from build123d import *

# Parameters (mm, degrees)
ESQUISSE2_W             = 35
ESQUISSE2_H             = 40
BOSS_EXTRU_1_DEPTH      = 5
ESQUISSE3_W             = 63
ESQUISSE3_H             = 38
BOSS_EXTRU_2_DEPTH      = 2.5
ENL_V_MAT_EXTRU_1_REACH = 58.932
ESQUISSE4_R             = 2
ENL_V_MAT_EXTRU_2_REACH = 58.932
ESQUISSE5_W             = 7
ESQUISSE5_H             = 18
CONG_1_R                = 2
CONG_2_R                = 5
CONG_3_R                = 2
ENL_V_MAT_EXTRU_3_REACH = 54.369
ESQUISSE6_R             = 2


with BuildPart() as part:
    # Esquisse2 → Boss.-Extru.1 (new body)
    with BuildSketch(Plane(origin=(0, 0, 0), x_dir=(1, 0, 0), z_dir=(0, 1, 0))):
        Rectangle(ESQUISSE2_W, ESQUISSE2_H)
    extrude(amount=BOSS_EXTRU_1_DEPTH)

    # Esquisse3 → Boss.-Extru.2 (add, symmetric)
    with BuildSketch(Plane(origin=(0, 0, 0), x_dir=(0, 0, -1), z_dir=(1, 0, 0))):
        with Locations((0, 24)):
            Rectangle(ESQUISSE3_W, ESQUISSE3_H)
    extrude(amount=BOSS_EXTRU_2_DEPTH, both=True)

    # Esquisse4 → Enlèv. mat.-Extru.1 (cut, up to next)
    with BuildSketch(Plane(origin=(2.5, 0, 0), x_dir=(0, 0, -1), z_dir=(1, 0, 0)), mode=Mode.PRIVATE) as enl_v_mat_extru_1_sk1:
        with Locations((-27.94, 37.97)):
            Circle(ESQUISSE4_R)
    enl_v_mat_extru_1_tool1 = extrude(enl_v_mat_extru_1_sk1.sketch, amount=-ENL_V_MAT_EXTRU_1_REACH, mode=Mode.PRIVATE) & part.part
    # Esquisse4 → Enlèv. mat.-Extru.1 (cut, up to next)
    with BuildSketch(Plane(origin=(2.5, 0, 0), x_dir=(0, 0, -1), z_dir=(1, 0, 0)), mode=Mode.PRIVATE) as enl_v_mat_extru_1_sk2:
        with Locations((-27.94, 10.03)):
            Circle(ESQUISSE4_R)
    enl_v_mat_extru_1_tool2 = extrude(enl_v_mat_extru_1_sk2.sketch, amount=-ENL_V_MAT_EXTRU_1_REACH, mode=Mode.PRIVATE) & part.part
    # Esquisse4 → Enlèv. mat.-Extru.1 (cut, up to next)
    with BuildSketch(Plane(origin=(2.5, 0, 0), x_dir=(0, 0, -1), z_dir=(1, 0, 0)), mode=Mode.PRIVATE) as enl_v_mat_extru_1_sk3:
        with Locations((27.94, 37.97)):
            Circle(ESQUISSE4_R)
    enl_v_mat_extru_1_tool3 = extrude(enl_v_mat_extru_1_sk3.sketch, amount=-ENL_V_MAT_EXTRU_1_REACH, mode=Mode.PRIVATE) & part.part
    # Esquisse4 → Enlèv. mat.-Extru.1 (cut, up to next)
    with BuildSketch(Plane(origin=(2.5, 0, 0), x_dir=(0, 0, -1), z_dir=(1, 0, 0)), mode=Mode.PRIVATE) as enl_v_mat_extru_1_sk4:
        with Locations((27.94, 10.03)):
            Circle(ESQUISSE4_R)
    enl_v_mat_extru_1_tool4 = extrude(enl_v_mat_extru_1_sk4.sketch, amount=-ENL_V_MAT_EXTRU_1_REACH, mode=Mode.PRIVATE) & part.part
    add(enl_v_mat_extru_1_tool1.solids().sort_by_distance((2.5, 37.97, 27.94))[0], mode=Mode.SUBTRACT)
    add(enl_v_mat_extru_1_tool2.solids().sort_by_distance((2.5, 10.03, 27.94))[0], mode=Mode.SUBTRACT)
    add(enl_v_mat_extru_1_tool3.solids().sort_by_distance((2.5, 37.97, -27.94))[0], mode=Mode.SUBTRACT)
    add(enl_v_mat_extru_1_tool4.solids().sort_by_distance((2.5, 10.03, -27.94))[0], mode=Mode.SUBTRACT)

    # Esquisse5 → Enlèv. mat.-Extru.2 (cut, up to next)
    with BuildSketch(Plane(origin=(2.5, 0, 0), x_dir=(0, 0, -1), z_dir=(1, 0, 0)), mode=Mode.PRIVATE) as enl_v_mat_extru_2_sk1:
        with Locations((-28, 24)):
            Rectangle(ESQUISSE5_W, ESQUISSE5_H)
    enl_v_mat_extru_2_tool1 = extrude(enl_v_mat_extru_2_sk1.sketch, amount=-ENL_V_MAT_EXTRU_2_REACH, mode=Mode.PRIVATE) & part.part
    # Esquisse5 → Enlèv. mat.-Extru.2 (cut, up to next)
    with BuildSketch(Plane(origin=(2.5, 0, 0), x_dir=(0, 0, -1), z_dir=(1, 0, 0)), mode=Mode.PRIVATE) as enl_v_mat_extru_2_sk2:
        with Locations((28, 24)):
            Rectangle(ESQUISSE5_W, ESQUISSE5_H)
    enl_v_mat_extru_2_tool2 = extrude(enl_v_mat_extru_2_sk2.sketch, amount=-ENL_V_MAT_EXTRU_2_REACH, mode=Mode.PRIVATE) & part.part
    add(enl_v_mat_extru_2_tool1.solids().sort_by_distance((2.5, 24, 28))[0], mode=Mode.SUBTRACT)
    add(enl_v_mat_extru_2_tool2.solids().sort_by_distance((2.5, 24, -28))[0], mode=Mode.SUBTRACT)

    # Congé1
    cong_1_edges = [part.edges().sort_by_distance(p)[0] for p in [
        (0, 15, -24.5),
        (0, 33, -24.5),
        (0, 15, 24.5),
        (0, 33, 24.5),
        (-2.5, 5, 0),
        (2.5, 5, 0),
    ]]
    fillet(cong_1_edges, radius=CONG_1_R)
    cong_1_2_edges = [part.edges().sort_by_distance(p)[0] for p in [
        (0, 5, -31.5),
        (0, 15, -31.5),
        (0, 43, -31.5),
        (0, 33, -31.5),
        (0, 5, 31.5),
        (0, 15, 31.5),
        (0, 33, 31.5),
        (0, 43, 31.5),
    ]]
    fillet(cong_1_2_edges, radius=CONG_1_R)

    # Congé2
    cong_2_edges = [part.edges().sort_by_distance(p)[0] for p in [
        (17.5, 2.5, 20),
        (-17.5, 2.5, 20),
        (-17.5, 2.5, -20),
        (17.5, 2.5, -20),
    ]]
    fillet(cong_2_edges, radius=CONG_2_R)

    # Congé3
    cong_3_edges = [part.edges().sort_by_distance(p)[0] for p in [
        (-2.5, 6, 20),
        (2.5, 6, 20),
        (0, 5, 20),
        (2.5, 6, -20),
        (-2.5, 6, -20),
        (0, 5, -20),
    ]]
    fillet(cong_3_edges, radius=CONG_3_R - 0.0001)  # a hair under: the kernel refuses the full size

    # Esquisse6 → Enlèv. mat.-Extru.3 (cut, up to next)
    with BuildSketch(Plane(origin=(0, 5, 0), x_dir=(1, 0, 0), z_dir=(0, 1, 0)), mode=Mode.PRIVATE) as enl_v_mat_extru_3_sk1:
        with Locations(Location((-11, 10, 0), (0, 0, 270))):
            Circle(ESQUISSE6_R)
    enl_v_mat_extru_3_tool1 = extrude(enl_v_mat_extru_3_sk1.sketch, amount=-ENL_V_MAT_EXTRU_3_REACH, mode=Mode.PRIVATE) & part.part
    # Esquisse6 → Enlèv. mat.-Extru.3 (cut, up to next)
    with BuildSketch(Plane(origin=(0, 5, 0), x_dir=(1, 0, 0), z_dir=(0, 1, 0)), mode=Mode.PRIVATE) as enl_v_mat_extru_3_sk2:
        with Locations(Location((-11, -10, 0), (0, 0, 270))):
            Circle(ESQUISSE6_R)
    enl_v_mat_extru_3_tool2 = extrude(enl_v_mat_extru_3_sk2.sketch, amount=-ENL_V_MAT_EXTRU_3_REACH, mode=Mode.PRIVATE) & part.part
    # Esquisse6 → Enlèv. mat.-Extru.3 (cut, up to next)
    with BuildSketch(Plane(origin=(0, 5, 0), x_dir=(1, 0, 0), z_dir=(0, 1, 0)), mode=Mode.PRIVATE) as enl_v_mat_extru_3_sk3:
        with Locations(Location((11, -10, 0), (0, 0, 90))):
            Circle(ESQUISSE6_R)
    enl_v_mat_extru_3_tool3 = extrude(enl_v_mat_extru_3_sk3.sketch, amount=-ENL_V_MAT_EXTRU_3_REACH, mode=Mode.PRIVATE) & part.part
    # Esquisse6 → Enlèv. mat.-Extru.3 (cut, up to next)
    with BuildSketch(Plane(origin=(0, 5, 0), x_dir=(1, 0, 0), z_dir=(0, 1, 0)), mode=Mode.PRIVATE) as enl_v_mat_extru_3_sk4:
        with Locations(Location((11, 10, 0), (0, 0, 90))):
            Circle(ESQUISSE6_R)
    enl_v_mat_extru_3_tool4 = extrude(enl_v_mat_extru_3_sk4.sketch, amount=-ENL_V_MAT_EXTRU_3_REACH, mode=Mode.PRIVATE) & part.part
    add(enl_v_mat_extru_3_tool1.solids().sort_by_distance((-11, 5, -10))[0], mode=Mode.SUBTRACT)
    add(enl_v_mat_extru_3_tool2.solids().sort_by_distance((-11, 5, 10))[0], mode=Mode.SUBTRACT)
    add(enl_v_mat_extru_3_tool3.solids().sort_by_distance((11, 5, 10))[0], mode=Mode.SUBTRACT)
    add(enl_v_mat_extru_3_tool4.solids().sort_by_distance((11, 5, -10))[0], mode=Mode.SUBTRACT)


solid = part.part
Geometry: final body of the model. Coordinates: model frame, mm. A direction names the side the tool comes from. Coordinates: 2 decimals unless noted, no trailing zeros. Order: outer loops, then holes, each group sorted by start corner. A loop starts at its lowest first (then second) coordinate and runs counter-clockwise, first axis right, second up. Notation, with made-up numbers: M -11,66 L 46,66 A11 cw 46,76 Z; hole C 40.25,19 d11. An arc over 180 degrees is marked long. One line per question, with ' | ' between items. Start each with the question number.
Item 1: Cut plane C-C, the plane x = -11. Return the cut outline in (y, z), then the cut area to 3 significant figures.
Item 2: Cut plane A-A, the plane y = 37.97. Return the cut outline in (x, z), then the cut area to 3 significant figures.
Item 3: Cut plane D-D, the plane z = 27.94. Return the cut outline in (x, y), then the cut area to 3 significant figures.
Item 4: Set-up query: faces 4 (the cylindrical face through (-0.04, 33.57, 30.9)), 5 (the flat face through (0, 15, -28)), 6 (the cylindrical face through (0.035, 37.204, -29.787)). Return all of +Z, -Z, +X, -X, +Y, -Y with unobstructed straight access to the full face (end or side cutting, diameter ignored); none if empty.
Item 5: Pin query (flat end, axial travel): pin 1 Ø5 at (x, z) = (11, -10) entering from +Y; pin 2 Ø5 at (x, z) = (-4.5, -24) entering from -Y; pin 3 Ø3 at (y, z) = (27.5, -24) entering from -X. Return the tip coordinate at first contact, or that it passes through.
Item 6: Draft query along Z for faces 1 (the flat face through (0, 5, 26)), 2 (the cylindrical face through (-16, 2.54, 18.57)), 3 (the cylindrical face through (9, 3, -10)). Return one class per face: released by +Z, released by -Z, zero draft, split by the parting line, or undercut.
Item 7: Ray query, probe 1 along X at (y, z) = (1.35, 10); probe 2 along Z at (x, y) = (11, 3.2); probe 3 along Y at (x, z) = (1.4, -27.94). Return the intervals inside material, ascending. Write a range as [from, to].
Item 8: Cut plane B-B, the plane z = -10. Return the cut outline in (x, y).
A:
1) outline: M 0,-20 L 5,-20 L 5,-12 L 0,-12 Z; M 0,-8 L 5,-8 L 5,8 L 0,8 Z; M 0,12 L 5,12 L 5,20 L 0,20 Z | area: 160 mm2
2) outline: M -2.5,-31.5 L 2.5,-31.5 L 2.5,-29.94 L -2.5,-29.94 Z; M -2.5,-25.94 L 2.5,-25.94 L 2.5,25.94 L -2.5,25.94 Z; M -2.5,29.94 L 2.5,29.94 L 2.5,31.5 L -2.5,31.5 Z | area: 275 mm2
3) outline: M -2.5,5 L 2.5,5 L 2.5,8.03 L -2.5,8.03 Z; M -2.5,12.03 L 2.5,12.03 L 2.5,15 L -2.5,15 Z; M -2.5,33 L 2.5,33 L 2.5,35.97 L -2.5,35.97 Z; M -2.5,39.97 L 2.5,39.97 L 2.5,43 L -2.5,43 Z | area: 60.0 mm2
4) face 4: +Z, +X, -X | face 5: -Z, +X, -X | face 6: +X, -X
5) pin 1: stops at y = 5 | pin 2: stops at y = 5 | pin 3: stops at x = -2.5
6) face 1: zero draft | face 2: released by +Z | face 3: undercut
7) probe 1: x = [-17.5, -13], [-9, 9], [13, 17.5] | probe 2: z = [-20, -12], [-8, 8], [12, 20] | probe 3: y = [5, 8.03], [12.03, 15], [33, 35.97], [39.97, 43]
8) outline: M -17.5,0 L -13,0 L -13,5 L -17.5,5 Z; M -9,0 L 9,0 L 9,5 L 4.5,5 A2 cw 2.5,7 L 2.5,43 L -2.5,43 L -2.5,7 A2 cw -4.5,5 L -9,5 Z; M 13,0 L 17.5,0 L 17.5,5 L 13,5 Z
